from build123d import *

# Parameters (mm, degrees)
PAD_DEPTH           = 3
PAD001_DEPTH        = 3
FILLET_R            = 3
FILLET001_R         = 1
FILLET002_R         = 1
SKETCH003_W         = 1.5
SKETCH003_H         = 14
SKETCH003_H_2       = 4
SKETCH003_W_2       = 40.5
SKETCH003_H_3       = 1.5
PAD002_DEPTH        = 1
SKETCH005_R         = 1.55
POCKET001_DEPTH     = 5
SKETCH004_W         = 2
SKETCH004_H         = 8
POCKET_DEPTH        = 4.001
LINEARPATTERN_COUNT = 5
LINEARPATTERN_PITCH = 3.4


with BuildPart() as part:
    # Sketch → Pad (new body)
    with BuildSketch(Plane.XY):
        Polygon((0, 3), (51, 3), (51, 0), (46.5, 0), (46.5, -20), (48.5, -20), (48.5, -36), (0, -36), align=None)
    extrude(amount=PAD_DEPTH)

    # Sketch001 (on Face10 of Pad) → Pad001 (join)
    with BuildSketch(Plane.XY.offset(3)):
        with BuildLine():
            Line((46.5, 6), (46.5, 3))
            Line((46.5, 3), (40.5, 3))
            Line((40.5, 3), (40.5, 6))
            ThreePointArc((46.5, 6), (43.5, 9), (40.5, 6))
        make_face()
    extrude(amount=-PAD001_DEPTH)

    # Fillet
    fillet_edges = [part.edges().sort_by_distance(p)[0] for p in [
        (48.5, -36, 1.5),
    ]]
    fillet(fillet_edges, radius=FILLET_R)

    # Fillet001
    fillet001_edges = [part.edges().sort_by_distance(p)[0] for p in [
        (48.5, -20, 1.5),
    ]]
    fillet(fillet001_edges, radius=FILLET001_R)

    # Fillet002
    fillet002_edges = [part.edges().sort_by_distance(p)[0] for p in [
        (51, 3, 1.5),
        (51, 0, 1.5),
    ]]
    fillet(fillet002_edges, radius=FILLET002_R)

    # Sketch003 → Pad002 (join)
    with BuildSketch(Plane(origin=(0, 0, 0), x_dir=(1, 0, 0), z_dir=(0, 0, -1))):
        with Locations((42.55, 9)):
            Rectangle(SKETCH003_W, SKETCH003_H)
        with Locations((44.55, 26)):
            Rectangle(SKETCH003_W, SKETCH003_H_2)
        with Locations((20.25, 32.05)):
            Rectangle(SKETCH003_W_2, SKETCH003_H_3)
    extrude(amount=PAD002_DEPTH)

    # Sketch005 (on Face28 of Pad002) → Pocket001 (cut)
    with BuildSketch(Plane.XY.offset(3)):
        with Locations((43.5, 6)):
            Circle(SKETCH005_R)
        with Locations((45.5, -33)):
            Circle(SKETCH005_R)
    extrude(amount=-POCKET001_DEPTH, mode=Mode.SUBTRACT)

    # Mirrored: part across YZ


with BuildPart() as part_1:
    add(part.part)
    add(part.part.mirror(Plane.YZ))

    # Sketch004 (on Face58 of Mirrored) → Pocket (cut, through all)
    with BuildSketch(Plane.XY.offset(3)):
        with Locations((32.5, -10.5)):
            Rectangle(SKETCH004_W, SKETCH004_H)
    pocket = extrude(amount=-POCKET_DEPTH, mode=Mode.SUBTRACT)

    # LinearPattern: Pocket ×5
    with Locations(*[(-i * LINEARPATTERN_PITCH, 0, 0) for i in range(1, LINEARPATTERN_COUNT)]):
        add(pocket, mode=Mode.SUBTRACT)


solid = part_1.part
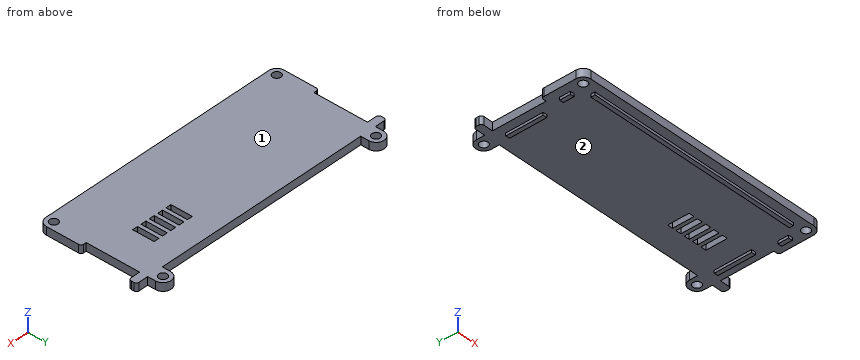
Check sheet for the modelled part. Datum: model origin and axes. Units: mm. Face numbers are marked on the shaded views. Give positions to 0.01 mm unless a question says otherwise; leave off trailing zeros. Write each loop counter-clockwise with the first axis right and the second up, starting at its lowest first coordinate (ties: lowest second). Pieces come first, ordered by that corner, then holes. Notation, with made-up numbers: (42, 46) -> (92, 46) arc R16 cw to (92, 75) -> close; hole circle Ø3 at (38, 44.25). An arc over 180 degrees is marked (long way). Use one line per item in the form item = value. Start each with the question number.
1. Section check C-C (x = 3). Record the cut outline in (y, z), and give its area (4 significant figures).
2. Section check B-B (y = -26). Record the cut outline in (x, z), and give its area (3 significant figures).
3. Mould release check, pull along X, two halves, no side actions. Record for the marked faces 1 and 2: pulls with the +X half, pulls with the -X half, needs draft (parallel to the pull), parting line crosses it, or undercut.
4. Section check A-A (y = -11). Count the separate pieces of the cut face and the enclosed holes in it, and give its area (3 significant figures).
5. Thickness scan on line 1 along Y through (x, z) = (-43.5, 1.9); line 2 along Y through (x, z) = (29.5, 0.6); line 3 along X through (y, z) = (-25.5, -0.6). Record the ranges inside material, lowest first. Write a range as from..to.
6. Go/stop test with flat-tipped pins: P1, Ø1.5, axis at y = -11, z = 1.5, coming from the -X side; P2, Ø0.5, axis at y = -26, z = -0.5, coming from the -X side; P3, Ø0.8, axis at y = -7, z = -0.5, coming from the -X side. Record where each tip stops, or that it passes through.
Conclusion:
q1.outline = (-36, 0) -> (-32.8, 0) -> (-32.8, -1) -> (-31.3, -1) -> (-31.3, 0) -> (3, 0) -> (3, 3) -> (-36, 3) -> close
q1.area = 118.5 mm²
q2.outline = (-48.5, 0) -> (-45.3, 0) -> (-45.3, -1) -> (-43.8, -1) -> (-43.8, 0) -> (43.8, 0) -> (43.8, -1) -> (45.3, -1) -> (45.3, 0) -> (48.5, 0) -> (48.5, 3) -> (-48.5, 3) -> close
q2.area = 294 mm²
q3.face_1 = needs draft
q3.face_2 = undercut
q4.separate_pieces = 6
q4.enclosed_holes = 0
q4.area = 252 mm²
q5.line_1 = -36..4.45, 7.55..9
q5.line_2 = -36..-14.5, -6.5..3
q5.line_3 = -45.3..-43.8, 43.8..45.3
q6.P1 = -46.5
q6.P2 = -45.3
q6.P3 = -43.3
